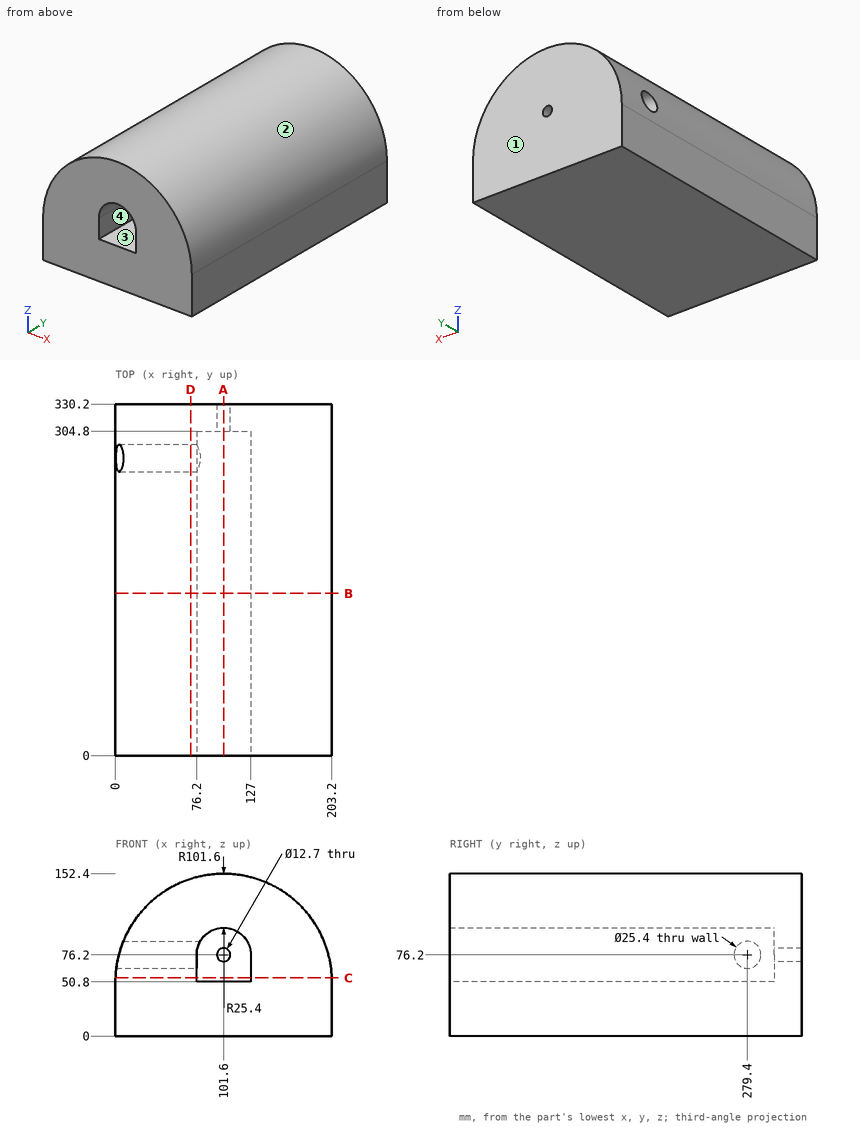
Could you check a few things on this drawing? It's one solid part, dimensions in mm from its lowest x, y, z. Round coordinates to 2 decimals unless told otherwise and drop trailing zeros. Write each loop counter-clockwise with the first axis right and the second up, starting at its lowest first coordinate (ties: lowest second). Pieces come first, ordered by that corner, then holes. Notation, with made-up numbers: M -30.5,65 L 12.5,65 A8 ccw 12.5,74 Z; hole C 5.25,44 d3. An arc over 180 degrees is marked long. Answer as CSV lines item,"result". Start each with the question number.
1. Suppose I cut it at B-B on y = 152.5. Write out the boundary of the cut face in (x, z), then the cut area to 3 significant figures.
2. Suppose I cut it at D-D on x = 70.5. Write out the boundary of the cut face in (y, z), then the cut area to 3 significant figures.
3. Suppose I cut it at A-A on x = 101.6. Write out the boundary of the cut face in (y, z), then the cut area to 3 significant figures.
4. Thinking about a two-plate mould opening in X: for the marked faces 1, 2, 3 and 4, which applies, released by +X, released by -X, zero draft, split by the parting line, or undercut?
5. I need wall thicknesses on probe 1 along Z at (x, y) = (101, 321); probe 2 along Y at (x, z) = (55, 76.2); probe 3 along Y at (x, z) = (50, 64.5). Which ranges of each line are inside material? Lowest first, please.
6. I'm going to push flat-ended pins straight in: pin 1 Ø1.5 at (y, z) = (97, 128) entering from +X; pin 2 Ø3 at (x, y) = (74, 198.5) entering from +Z; pin 3 Ø7.5 at (y, z) = (186.5, 68.5) entering from +X. Where does each tip first touch, or does it pass through?
7. Suppose I cut it at C-C on z = 54.5. Write out the boundary of the cut face in (x, y).
Check result:
1,outline,"M 0,0 L 203.2,0 L 203.2,50.8 A101.6 ccw 0,50.8 Z; hole M 76.2,50.8 L 127,50.8 L 127,76.2 A25.4 ccw 76.2,76.2 Z"
1,area,"24,200 mm2"
2,outline,"M 0,0 L 330.2,0 L 330.2,147.52 L 0,147.52 Z; hole C 279.4,76.2 d25.4"
2,area,"48,200 mm2"
3,outline,"M 0,0 L 330.2,0 L 330.2,69.85 L 304.8,69.85 L 304.8,50.8 L 0,50.8 Z; M 0,101.6 L 304.8,101.6 L 304.8,82.55 L 330.2,82.55 L 330.2,152.4 L 0,152.4 Z"
3,area,"34,500 mm2"
4,face 1,"zero draft"
4,face 2,"split by the parting line"
4,face 3,"undercut"
4,face 4,"undercut"
5,probe 1,"z = 0 to 69.88, 82.52 to 152.4"
5,probe 2,"y = 0 to 266.7, 292.1 to 330.2"
5,probe 3,"y = 0 to 274.46, 284.34 to 330.2"
6,pin 1,"stops at x = 168.52"
6,pin 2,"stops at z = 148.99"
6,pin 3,"stops at x = 202.24"
7,outline,"M 0.07,0 L 76.2,0 L 76.2,304.8 L 127,304.8 L 127,0 L 203.13,0 L 203.13,330.2 L 0.07,330.2 Z"
